Can you work these out from the drawing? Everything is in mm from the part's minimum corner. A direction names the side the tool comes from. Coordinates: 2 decimals unless noted, no trailing zeros. Write each loop counter-clockwise with the first axis right and the second up, starting at its lowest first coordinate (ties: lowest second). Pieces come first, ordered by that corner, then holes.
(1) Imagine slicing it at D-D, the plane z = 10.25. List the corners of the cut face in (x, y) for me, plus the area to 3 significant figures.
(2) Which directions (+Z, -Z, +X, -X, +Y, -Y) give clear straight access to the entire face, cutting with the end or side of a thin tool? Please do the marked faces 4 and 5.
(3) Imagine slicing it at B-B, the plane x = 22.5. List the corners of the cut face in (y, z) for me, plus the area to 3 significant figures.
(4) Thinking about a two-plate mould opening in X: for the marked faces 1, 2 and 3, which applies, released by +X, released by -X, zero draft, split by the parting line, or undercut?
(5) Imagine slicing it at C-C, the plane y = 23.5. List the corners of the cut face in (x, z) for me.
(6) Imagine slicing it at A-A, the plane y = 13. List the corners of the cut face in (x, z) for me, plus the area to 3 significant figures.
(7) Please list where these lines run through material, in increasing order: probe 1 along Y at (x, z) = (10, 9.25); probe 2 along X at (y, z) = (7.5, 9.25); probe 3 along Y at (x, z) = (13, 0.5).
(8) For pin 1 Ø1.6 at (x, z) = (1.5, 7) entering from -Y; pin 2 Ø2 at (x, y) = (8, 32.5) entering from +Z; pin 3 Ø1 at (x, z) = (1, 6.5) entering from +Y, each with a flat end and sliding along its axis, tell me the tip position at first contact or that it passes through.
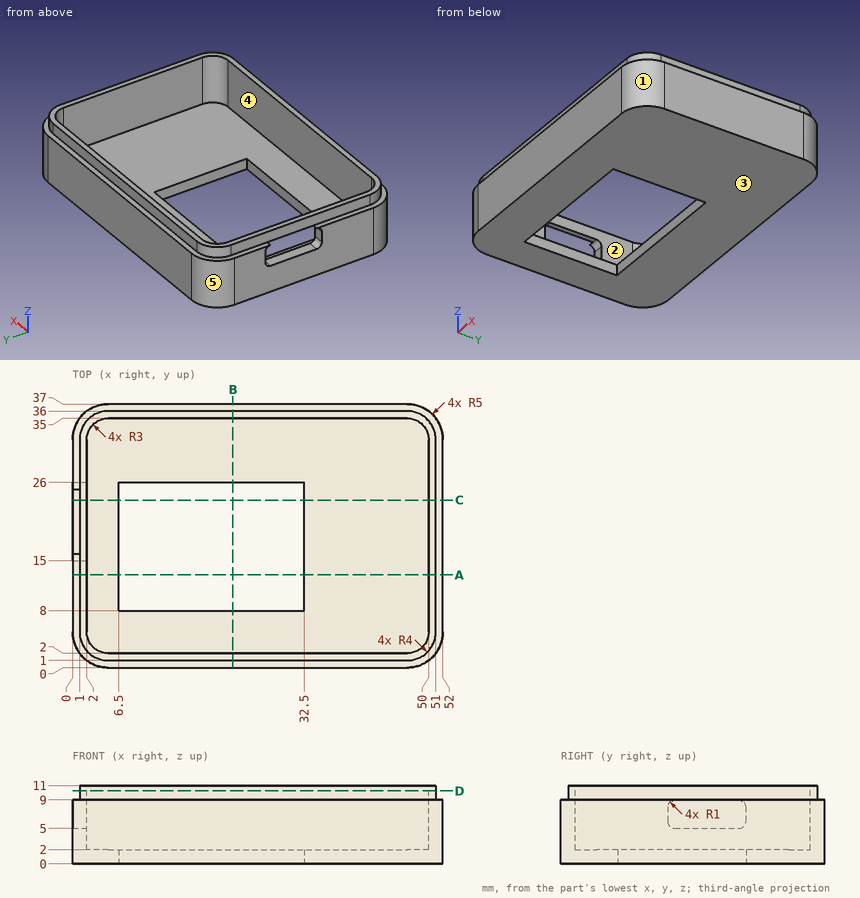
Recorded:
1. outline: (1, 5) arc R4 ccw to (5, 1) - (47, 1) arc R4 ccw to (51, 5) - (51, 32) arc R4 ccw to (47, 36) - (5, 36) arc R4 ccw to (1, 32) - close; hole (2, 5) arc R3 ccw to (5, 2) - (47, 2) arc R3 ccw to (50, 5) - (50, 32) arc R3 ccw to (47, 35) - (5, 35) arc R3 ccw to (2, 32) - close
1. area: 160 mm2
2. face 4: +Z
2. face 5: +Z, -Z, -X, +Y
3. outline: (0, 0) - (8, 0) - (8, 2) - (2, 2) - (2, 11) - (1, 11) - (1, 9) - (0, 9) - close; (26, 0) - (37, 0) - (37, 9) - (36, 9) - (36, 11) - (35, 11) - (35, 2) - (26, 2) - close
3. area: 70.0 mm2
4. face 1: released by +X
4. face 2: undercut
4. face 3: zero draft
5. outline: (0, 0) - (6.5, 0) - (6.5, 2) - (2, 2) - (2, 5) - (0, 5) - close; (1, 9) - (2, 9) - (2, 11) - (1, 11) - close; (32.5, 0) - (52, 0) - (52, 9) - (51, 9) - (51, 11) - (50, 11) - (50, 2) - (32.5, 2) - close
6. outline: (0, 0) - (6.5, 0) - (6.5, 2) - (2, 2) - (2, 11) - (1, 11) - (1, 9) - (0, 9) - close; (32.5, 0) - (52, 0) - (52, 9) - (51, 9) - (51, 11) - (50, 11) - (50, 2) - (32.5, 2) - close
6. area: 84.0 mm2
7. probe 1: y = 1 to 2, 35 to 36
7. probe 2: x = 1 to 2, 50 to 51
7. probe 3: y = 0 to 8, 26 to 37
8. pin 1: stops at y = 0.79
8. pin 2: stops at z = 2
8. pin 3: stops at y = 35.57
